CAD build for the part. Positions are in the model's coordinates, mm. Give positions to 0.01 mm unless a question says otherwise; leave off trailing zeros. Order: outer loops, then holes, each group sorted by start corner. A loop starts at its lowest first (then second) coordinate and runs counter-clockwise, first axis right, second up. Notation, with made-up numbers: (29.25, 13.5) -> (87.25, 13.5) arc R20 ccw to (87.25, 50.5) -> close; hole circle Ø9 at (21, -18). An arc over 180 degrees is marked (long way). Use one line per item in the form item = value. Start each with the question number.
1) Cut at A-A, the plane x = -32. Give the cut face in (y, z).
2) Drop flat-ended pins along their axis: P1, Ø1.5, axis at x = -29, z = 2, coming from the -Y side; P2, Ø1, axis at x = -45, z = 2, coming from the +Y side; P3, Ø13, axis at x = -32.3, y = 116.58, coming from the +Z side. Give the stop position or say it passes through.
3) Cut at C-C, the plane x = -38. Give the cut face in (y, z), and give its area (3 significant figures).
4) Probe line 1 (X direction, y = 120.5, z = 1.5); line 2 (X direction, y = 91, z = 0.75); line 3 (Y direction, x = -57, z = 2.95). List the from-to ranges inside material, lowest first.
5) Cut at D-D, the plane z = 0.9. State how many separate pieces and enclosed holes the cut face has, and give its area (3 significant figures).
6) Cut at B-B, the plane y = 90.5. Give the cut face in (x, z), and give its area (3 significant figures).
7) Mould opens along X. For faces 1 (the face through (-41.38, 100.73, 1.48)), 2 (the face through (-33.386, 121.486, 1.479)), 3 (the face through (-62.53, 96.89, 1.48)) say: pulls with the +X half, pulls with the -X half, needs draft (parallel to the pull), parting line crosses it, or undercut.
Autodesk Inventor part; units mm, degrees
ref_plane "YZ Plane" through (0, 0, 0) normal (1, 0, 0) x (0, 1, 0)
ref_plane "XZ Plane" through (0, 0, 0) normal (0, 1, 0) x (-1, 0, 0)
ref_plane "XY Plane" through (0, 0, 0) normal (0, 0, 1) x (1, 0, 0)
sketch "スケッチ2" plane through (0, 0, 0) normal (0, 0, 1) x (1, 0, 0)
  circle A0 centre (-56.644, 91.4364) radius 8.025
  circle A1 centre (-56.644, 91.4364) radius 5.025
  arc A2 (-29.1424, 109.2011) -> (-49.1672, 88.5212) centre (-14.5297, 75.0161) ccw
  arc A3 (-59.7983, 98.8155) -> (-39.7735, 119.4954) centre (-74.411, 133.0005) ccw
  circle A4 centre (-32.2967, 116.5802) radius 8.025
  circle A5 centre (-32.2967, 116.5802) radius 5.025
  line L0 (-50.8789, 85.8539) -> (-64.3562, 71.9357)
  line L1 (-64.3562, 71.9357) -> (-64.668, 91.3073)
  line L2 (-56.644, 91.4364) -> (-32.2967, 116.5802) construction
  point P0 (0, 0)
  point P1 (0, 0)
  dimension "d5" = 45
extrude "押し出し2" add sketch "スケッチ2" along normal blind 3
fillet "フィレット2" radius 0.5 1 edges at (-64.3562, 71.9357, 1.5)
sketch "スケッチ3" plane through (0, 0, 3) normal (0, 0, 1) x (1, 0, 0)
  line L0 (-63.5165, 72.8029) -> (-50.8789, 85.8539)
  arc A0 (-64.3756, 73.1427) -> (-63.5165, 72.8029) centre (-63.8757, 73.1507) ccw
  line L1 (-64.668, 91.3073) -> (-64.3756, 73.1427)
  arc A1 (-59.7983, 98.8155) -> (-64.668, 91.3073) centre (-56.644, 91.4364) ccw
  circle A2 centre (-56.644, 91.4364) radius 5.025
  arc A3 (-50.8789, 85.8539) -> (-49.1672, 88.5212) centre (-56.644, 91.4364) ccw
  line L2 (-64.2129, 94.1033) -> (-63.8416, 71.0319)
  point P0 (0, 0)
  point P1 (-63.8676, 72.6508)
  dimension "d9" = 0.5
extrude "押し出し3" cut sketch "スケッチ3" against normal through all
fillet "フィレット3" radius 1 1 edges at (-63.8676, 72.6508, 1.5)
properties part number "アーム揺動節2" material "アルミニウム 2014-T4"
Result:
q1.outline = (107.83, 0) -> (111.56, 0) -> (111.56, 3) -> (107.83, 3) -> close; (121.6, 0) -> (124.6, 0) -> (124.6, 3) -> (121.6, 3) -> close
q2.P1 = 108.93
q2.P2 = 110.92
q2.P3 = 3
q3.outline = (103.85, 0) -> (122.23, 0) -> (122.23, 3) -> (103.85, 3) -> close
q3.area = 55.1 mm²
q4.line_1 = -39.3 to -35.44, -29.15 to -25.29
q4.line_2 = -64.16 to -61.65, -51.64 to -48.1
q4.line_3 = 79.53 to 86.42, 96.45 to 100.15
q5.separate_pieces = 1
q5.enclosed_holes = 2
q5.area = 523 mm²
q6.outline = (-64.15, 0) -> (-61.58, 0) -> (-61.58, 3) -> (-64.15, 3) -> close; (-51.71, 0) -> (-48.33, 0) -> (-48.33, 3) -> (-51.71, 3) -> close
q6.area = 17.9 mm²
q7.face_1 = pulls with the +X half
q7.face_2 = undercut
q7.face_3 = pulls with the -X half
